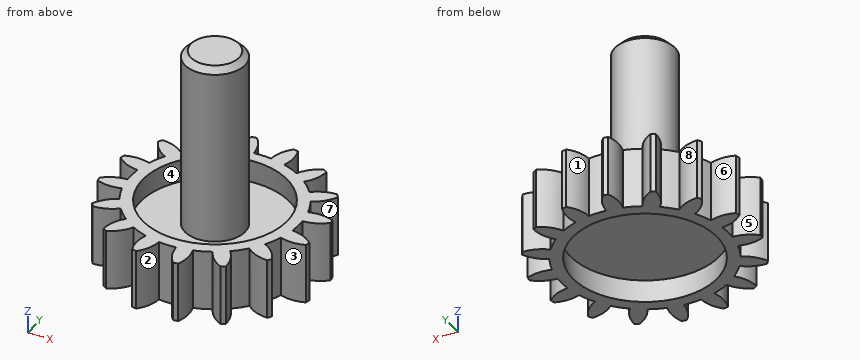
```python
from build123d import *

# Parameters (mm, degrees)
SKETCH_1_R          = 18
EXTRUDE_1_DEPTH     = 10
CUT_EXTRUDE_2_DEPTH = 28.349588662
SKETCH_4_R          = 12
CUT_EXTRUDE_3_DEPTH = 4
CUT_EXTRUDE_3_DRAFT = 6
SKETCH_5_R          = 5
EXTRUDE_2_DEPTH     = 30
CHAMFER_1_SIZE      = 1
SKETCH_6_R          = 12
CUT_EXTRUDE_4_DEPTH = 4
CUT_EXTRUDE_4_DRAFT = 6


with BuildPart() as part:
    # Эскиз1 → Бобышка-Вытянуть1 (new body)
    with BuildSketch(Plane.XY):
        Circle(SKETCH_1_R)
    extrude(amount=-EXTRUDE_1_DEPTH)

    # Эскиз3 → Вырез-Вытянуть2 (cut, through all)
    with BuildSketch(Plane.XY):
        with BuildLine():
            ThreePointArc((1.463398486, 13.923306535), (0, 14), (-1.463398486, 13.923306535))
            ThreePointArc((-1.463398486, 13.923306535), (-1.955189123, 15.973239081), (-3.125667198, 17.726539554))
            ThreePointArc((-3.125667198, 17.726539554), (0, 18), (3.125667198, 17.726539554))
            ThreePointArc((3.125667198, 17.726539554), (1.955189123, 15.973239081), (1.463398486, 13.923306535))
        make_face()
        with BuildLine():
            ThreePointArc((6.680222644, 12.303439577), (5.357568053, 12.934313455), (3.976214826, 13.423476288))
            ThreePointArc((3.976214826, 13.423476288), (4.306334745, 15.505567139), (3.895913051, 17.573328128))
            ThreePointArc((3.895913051, 17.573328128), (6.888301783, 16.629831585), (9.67139295, 15.181046025))
            ThreePointArc((9.67139295, 15.181046025), (7.91905317, 14.009130171), (6.680222644, 12.303439577))
        make_face()
        with BuildLine():
            ThreePointArc((10.88004346, 8.810485475), (9.899494937, 9.899494937), (8.810485475, 10.88004346))
            ThreePointArc((8.810485475, 10.88004346), (9.912258185, 12.677313159), (10.324375854, 14.744736797))
            ThreePointArc((10.324375854, 14.744736797), (12.727922061, 12.727922061), (14.744736797, 10.324375854))
            ThreePointArc((14.744736797, 10.324375854), (12.677313159, 9.912258185), (10.88004346, 8.810485475))
        make_face()
        with BuildLine():
            ThreePointArc((13.423476288, 3.976214826), (12.934313455, 5.357568053), (12.303439577, 6.680222644))
            ThreePointArc((12.303439577, 6.680222644), (14.009130171, 7.91905317), (15.181046025, 9.67139295))
            ThreePointArc((15.181046025, 9.67139295), (16.629831585, 6.888301783), (17.573328128, 3.895913051))
            ThreePointArc((17.573328128, 3.895913051), (15.505567139, 4.306334745), (13.423476288, 3.976214826))
        make_face()
        with BuildLine():
            ThreePointArc((13.923306535, -1.463398486), (14, 0), (13.923306535, 1.463398486))
            ThreePointArc((13.923306535, 1.463398486), (15.973239081, 1.955189123), (17.726539554, 3.125667198))
            ThreePointArc((17.726539554, 3.125667198), (18, 0), (17.726539554, -3.125667198))
            ThreePointArc((17.726539554, -3.125667198), (15.973239081, -1.955189123), (13.923306535, -1.463398486))
        make_face()
        with BuildLine():
            ThreePointArc((12.303439577, -6.680222644), (12.934313455, -5.357568053), (13.423476288, -3.976214826))
            ThreePointArc((13.423476288, -3.976214826), (15.505567139, -4.306334745), (17.573328128, -3.895913051))
            ThreePointArc((17.573328128, -3.895913051), (16.629831585, -6.888301783), (15.181046025, -9.67139295))
            ThreePointArc((15.181046025, -9.67139295), (14.009130171, -7.91905317), (12.303439577, -6.680222644))
        make_face()
        with BuildLine():
            ThreePointArc((8.810485475, -10.88004346), (9.899494937, -9.899494937), (10.88004346, -8.810485475))
            ThreePointArc((10.88004346, -8.810485475), (12.677313159, -9.912258185), (14.744736797, -10.324375854))
            ThreePointArc((14.744736797, -10.324375854), (12.727922061, -12.727922061), (10.324375854, -14.744736797))
            ThreePointArc((10.324375854, -14.744736797), (9.912258185, -12.677313159), (8.810485475, -10.88004346))
        make_face()
        with BuildLine():
            ThreePointArc((3.976214826, -13.423476288), (5.357568053, -12.934313455), (6.680222644, -12.303439577))
            ThreePointArc((6.680222644, -12.303439577), (7.91905317, -14.009130171), (9.67139295, -15.181046025))
            ThreePointArc((9.67139295, -15.181046025), (6.888301783, -16.629831585), (3.895913051, -17.573328128))
            ThreePointArc((3.895913051, -17.573328128), (4.306334745, -15.505567139), (3.976214826, -13.423476288))
        make_face()
        with BuildLine():
            ThreePointArc((-1.463398486, -13.923306535), (0, -14), (1.463398486, -13.923306535))
            ThreePointArc((1.463398486, -13.923306535), (1.955189123, -15.973239081), (3.125667198, -17.726539554))
            ThreePointArc((3.125667198, -17.726539554), (0, -18), (-3.125667198, -17.726539554))
            ThreePointArc((-3.125667198, -17.726539554), (-1.955189123, -15.973239081), (-1.463398486, -13.923306535))
        make_face()
        with BuildLine():
            ThreePointArc((-6.680222644, -12.303439577), (-5.357568053, -12.934313455), (-3.976214826, -13.423476288))
            ThreePointArc((-3.976214826, -13.423476288), (-4.306334745, -15.505567139), (-3.895913051, -17.573328128))
            ThreePointArc((-3.895913051, -17.573328128), (-6.888301783, -16.629831585), (-9.67139295, -15.181046025))
            ThreePointArc((-9.67139295, -15.181046025), (-7.91905317, -14.009130171), (-6.680222644, -12.303439577))
        make_face()
        with BuildLine():
            ThreePointArc((-10.88004346, -8.810485475), (-9.899494937, -9.899494937), (-8.810485475, -10.88004346))
            ThreePointArc((-8.810485475, -10.88004346), (-9.912258185, -12.677313159), (-10.324375854, -14.744736797))
            ThreePointArc((-10.324375854, -14.744736797), (-12.727922061, -12.727922061), (-14.744736797, -10.324375854))
            ThreePointArc((-14.744736797, -10.324375854), (-12.677313159, -9.912258185), (-10.88004346, -8.810485475))
        make_face()
        with BuildLine():
            ThreePointArc((-13.423476288, -3.976214826), (-12.934313455, -5.357568053), (-12.303439577, -6.680222644))
            ThreePointArc((-12.303439577, -6.680222644), (-14.009130171, -7.91905317), (-15.181046025, -9.67139295))
            ThreePointArc((-15.181046025, -9.67139295), (-16.629831585, -6.888301783), (-17.573328128, -3.895913051))
            ThreePointArc((-17.573328128, -3.895913051), (-15.505567139, -4.306334745), (-13.423476288, -3.976214826))
        make_face()
        with BuildLine():
            ThreePointArc((-13.923306535, 1.463398486), (-14, 0), (-13.923306535, -1.463398486))
            ThreePointArc((-13.923306535, -1.463398486), (-15.973239081, -1.955189123), (-17.726539554, -3.125667198))
            ThreePointArc((-17.726539554, -3.125667198), (-18, 0), (-17.726539554, 3.125667198))
            ThreePointArc((-17.726539554, 3.125667198), (-15.973239081, 1.955189123), (-13.923306535, 1.463398486))
        make_face()
        with BuildLine():
            ThreePointArc((-12.303439577, 6.680222644), (-12.934313455, 5.357568053), (-13.423476288, 3.976214826))
            ThreePointArc((-13.423476288, 3.976214826), (-15.505567139, 4.306334745), (-17.573328128, 3.895913051))
            ThreePointArc((-17.573328128, 3.895913051), (-16.629831585, 6.888301783), (-15.181046025, 9.67139295))
            ThreePointArc((-15.181046025, 9.67139295), (-14.009130171, 7.91905317), (-12.303439577, 6.680222644))
        make_face()
        with BuildLine():
            ThreePointArc((-8.810485475, 10.88004346), (-9.899494937, 9.899494937), (-10.88004346, 8.810485475))
            ThreePointArc((-10.88004346, 8.810485475), (-12.677313159, 9.912258185), (-14.744736797, 10.324375854))
            ThreePointArc((-14.744736797, 10.324375854), (-12.727922061, 12.727922061), (-10.324375854, 14.744736797))
            ThreePointArc((-10.324375854, 14.744736797), (-9.912258185, 12.677313159), (-8.810485475, 10.88004346))
        make_face()
        with BuildLine():
            ThreePointArc((-3.976214826, 13.423476288), (-5.357568053, 12.934313455), (-6.680222644, 12.303439577))
            ThreePointArc((-6.680222644, 12.303439577), (-7.91905317, 14.009130171), (-9.67139295, 15.181046025))
            ThreePointArc((-9.67139295, 15.181046025), (-6.888301783, 16.629831585), (-3.895913051, 17.573328128))
            ThreePointArc((-3.895913051, 17.573328128), (-4.306334745, 15.505567139), (-3.976214826, 13.423476288))
        make_face()
    extrude(amount=-CUT_EXTRUDE_2_DEPTH, mode=Mode.SUBTRACT)


with BuildPart() as cut_extrude_3_tool:
    # Эскиз4 → Вырез-Вытянуть3 (with draft: the straight prism first)
    with BuildSketch(Plane.XY):
        Circle(SKETCH_4_R)
    extrude(amount=-CUT_EXTRUDE_3_DEPTH)
    # Вырез-Вытянуть3: the draft: its side faces are tilted about the plane it starts from
    cut_extrude_3_sides = [cut_extrude_3_tool.faces().sort_by_distance(p)[0] for p in [
        (-12, 0, -2),
    ]]
    draft(cut_extrude_3_sides, Plane.XY, CUT_EXTRUDE_3_DRAFT)


with BuildPart() as part_1:
    add(part.part)

    # Вырез-Вытянуть3: cut by cut_extrude_3_tool
    add(cut_extrude_3_tool.part, mode=Mode.SUBTRACT)

    # Эскиз5 → Бобышка-Вытянуть2 (add)
    with BuildSketch(Plane.XY.offset(-4)):
        Circle(SKETCH_5_R)
    extrude(amount=EXTRUDE_2_DEPTH)

    # Фаска1
    chamfer_1_edges = [part_1.edges().sort_by_distance(p)[0] for p in [
        (-5, 0, 26),
    ]]
    chamfer(chamfer_1_edges, length=CHAMFER_1_SIZE)


with BuildPart() as cut_extrude_4_tool:
    # Эскиз6 → Вырез-Вытянуть4 (with draft: the straight prism first)
    with BuildSketch(Plane(origin=(0, 0, -10), x_dir=(-1, 0, 0), z_dir=(0, 0, -1))):
        Circle(SKETCH_6_R)
    extrude(amount=-CUT_EXTRUDE_4_DEPTH)
    # Вырез-Вытянуть4: the draft: its side faces are tilted about the plane it starts from
    cut_extrude_4_sides = [cut_extrude_4_tool.faces().sort_by_distance(p)[0] for p in [
        (12, 0, -8),
    ]]
    draft(cut_extrude_4_sides, Plane(origin=(0, 0, -10), x_dir=(-1, 0, 0), z_dir=(0, 0, -1)), CUT_EXTRUDE_4_DRAFT)


with BuildPart() as part_2:
    add(part_1.part)

    # Вырез-Вытянуть4: cut by cut_extrude_4_tool
    add(cut_extrude_4_tool.part, mode=Mode.SUBTRACT)


solid = part_2.part
```
The listing builds one solid part. Answer for the finished solid, in the listing's coordinates (mm). Face numbers are marked on the shaded views. A direction names the side the tool comes from. Coordinates: 2 decimals unless noted, no trailing zeros. Write each loop counter-clockwise with the first axis right and the second up, starting at its lowest first coordinate (ties: lowest second). Pieces come first, ordered by that corner, then holes. Notation, with made-up numbers: (17.5, 23) - (38.5, 23) arc R24 cw to (38.5, 39) - close; hole circle Ø4 at (80.25, 15). An arc over 180 degrees is marked (long way). Return JSON: item names as keys, results as strings. Group by question number.
1. Straight lines are drawn through the part: L1, parallel to Y at x = 14.5, z = -1; L2, parallel to Y at x = -15, z = -1.5; L3, parallel to X at y = -3.5, z = -2. For each, find the intervals that lie inside material, in ascending order.
2. A cutting plane is placed at A-A, the plane y = 0. Determine the outline of the cut face in (x, z), plus the area to 3 significant figures.
3. Given pin 1 (10 mm diameter, centred on y = 4, z = 9.5, fed in from -X); pin 2 (5 mm diameter, centred on x = 0, z = -4, fed in from -Y); pin 3 (10 mm diameter, centred on x = 0, y = -5.5, fed in from -Z), each flat-ended and moving along its own axis, determine where each tip first touches the part or whether it passes through.
4. Determine the mould class of the marked faces 5, 6, 7 and 8 for opening direction X: released by +X, released by -X, zero draft, split by the parting line, or undercut.
5. A cutting plane is placed at C-C, the plane z = 19.5. Determine the outline of the cut face in (x, y), plus the area to 3 significant figures.
6. Which of the six approach directions +Z, -Z, +X, -X, +Y, -Y give full straight-line access (tool end or side, diameter ignored) to the marked faces 1, 2, 3 and 4?
Ans:
{
 "1": {"L1": "-10.31 to -8.5, -4.24 to -1.53, 1.53 to 4.24, 8.5 to 10.31", "L2": "-9.95 to -9.29, -4.29 to -1.63, 1.63 to 4.29, 9.29 to 9.95", "L3": "-17.66 to -11.7, -3.57 to 3.57, 11.7 to 17.66"},
 "2": {"outline": "(-14, -10) - (-12, -10) - (-12.42, -6) - (12.42, -6) - (12, -10) - (14, -10) - (14, 0) - (12, 0) - (12.42, -4) - (5, -4) - (5, 25) - (4, 26) - (-4, 26) - (-5, 25) - (-5, -4) - (-12.42, -4) - (-12, 0) - (-14, 0) - close", "area": "384 mm²"},
 "3": {"pin 1": "x = -5", "pin 2": "y = -16.96", "pin 3": "z = -6"},
 "4": {"face 5": "released by -X", "face 6": "undercut", "face 7": "released by +X", "face 8": "undercut"},
 "5": {"outline": "circle Ø10 at (0, 0)", "area": "78.5 mm²"},
 "6": {"face 1": "+Z, -Z, +Y", "face 2": "+Z, -Z, -Y", "face 3": "+Z, -Z", "face 4": "none"}
}
